Autodesk Inventor part; units mm, degrees
ref_plane "YZ Plane" through (0, 0, 0) normal (1, 0, 0) x (0, 1, 0)
ref_plane "XZ Plane" through (0, 0, 0) normal (0, 1, 0) x (-1, 0, 0)
ref_plane "XY Plane" through (0, 0, 0) normal (0, 0, 1) x (1, 0, 0)
sketch "Sketch1" plane through (0, 0, 0) normal (0, 0, 1) x (1, 0, 0)
  line L0 (-46.9696, 22.7927) -> (33.4304, 22.7927)
  line L1 (33.4304, 22.7927) -> (33.4304, -14.6073)
  line L2 (33.4304, -14.6073) -> (-46.9696, -14.6073)
  line L3 (-46.9696, -14.6073) -> (-46.9696, 22.7927)
  circle A0 centre (-44.4696, 20.2927) radius 1
  circle A1 centre (-44.4696, -12.1073) radius 1
  circle A2 centre (30.9304, -12.1073) radius 1
  circle A3 centre (30.9304, 20.2927) radius 1
  point P0 (0, 0)
  dimension "d0" = 80.4
  dimension "d1" = 37.4
  dimension "d2" = 75.4
  dimension "d3" = 32.4
  dimension "d4" = 32.4
  dimension "d5" = 75.4
  dimension "d6" = 2.5
  dimension "d7" = 2.5
  dimension "d8" = 2
  dimension "d9" = 2
  dimension "d10" = 2
  dimension "d11" = 2
extrude "Extrusion1" add sketch "Sketch1" along normal blind 2
sketch "Sketch2" plane through (0, 0, 2) normal (0, 0, 1) x (1, 0, 0)
  circle A0 centre (-44.4696, 20.2927) radius 1
  circle A1 centre (-44.4696, -12.1073) radius 1
  circle A2 centre (30.9304, -12.1073) radius 1
  circle A3 centre (30.9304, 20.2927) radius 1
  point P0 (0, 0)
hole "Hole1" at (-44.4696, 20.2927, 2) at (-44.4696, -12.1073, 2) at (30.9304, -12.1073, 2) at (30.9304, 20.2927, 2) direction (0, 0, -1) diameter 2 depth 8 tip angle 118 countersink diameter 5 countersink angle 90
properties part number "case cover"
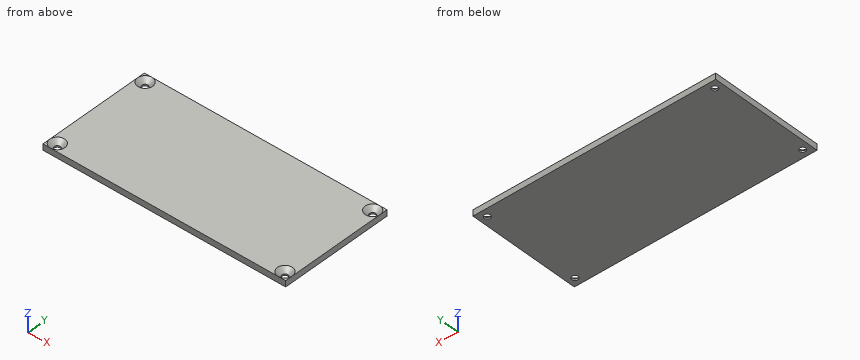
The model under review builds one solid part; all positions refer to its coordinate system, in mm. Round coordinates to 2 decimals unless told otherwise and drop trailing zeros. Order: outer loops, then holes, each group sorted by start corner. A loop starts at its lowest first (then second) coordinate and runs counter-clockwise, first axis right, second up. Notation, with made-up numbers: (0, -40) -> (43, -40) arc R23 ccw to (43, -21) -> close; hole circle Ø8 at (-13.75, 61.25). An arc over 180 degrees is marked (long way). Write item = value, one per line. Start each with the question number.
Item 1: For line 1 along X through (y, z) = (-12, 1.1); line 2 along X through (y, z) = (19, 0.95), list the stretches that pass through material, from the lowest coordinate up.
Item 2: Clearance check with a flat-ended pin moving along its axis: pin 1 Ø2.5 at (x, y) = (-44.47, -12.11) entering from +Z. State where the tip first meets the part, or that it passes through.
Item 3: Consider section A-A on z = 1.4. Write out the cut boundary in (x, y), plus the area to 3 significant figures.
Conclusion:
q1.line_1 = -46.97 to -46.07, -42.87 to 29.33, 32.53 to 33.43
q1.line_2 = -46.97 to -45.13, -43.81 to 30.27, 31.59 to 33.43
q2.pin_1 = 0.75
q3.outline = (-46.97, -14.61) -> (33.43, -14.61) -> (33.43, 22.79) -> (-46.97, 22.79) -> close; hole circle Ø3.8 at (-44.47, -12.11); hole circle Ø3.8 at (-44.47, 20.29); hole circle Ø3.8 at (30.93, -12.11); hole circle Ø3.8 at (30.93, 20.29)
q3.area = 2,960 mm2
